For this review, take the finished solid that the model builds, in its own axes (mm). A direction names the side the tool comes from. Round coordinates to 2 decimals unless told otherwise and drop trailing zeros. Loops run counter-clockwise (first coordinate to the right, second up) from the corner with the lowest first, then second, coordinate; pieces in that order, holes last.
1) Take a section at A-A (z = -36). State the section outline as (x, y) points, then the cut area to 3 significant figures.
2) Mouldability with a two-part tool opening along X and no side actions: class faces 3 (the cylindrical face through (23.43, 1.52, -0.6)), 4 (the cylindrical face through (7.95, 1.52, -28.06)), 5 (the flat face through (6, 0, -45)) as pulls with the +X half, pulls with the -X half, needs draft (parallel to the pull), parting line crosses it, or undercut.
3) Take a section at C-C (x = 11). State the section outline as (y, z) points, then the cut area to 3 significant figures.
4) Wall thickness on L1, parallel to X at y = 0.8, z = -68; L2, parallel to X at y = 0.95, z = -84; L3, parallel to Z at x = 13.5, y = 1.45: over which ranges is each line inside the solid? List them lowest first.
5) Take a section at D-D (y = 1.85). Give the number of separate pieces and of enclosed holes in the cut face, then the cut area to 3 significant figures.
6) Tool access review of faces 1 (the cylindrical face through (16.05, 1.52, -43.94)), 2 (the flat face through (12, 1, -88)): name each direction out of +Z, -Z, +X, -X, +Y, -Y from which nothing blocks a thin tool from reaching the whole face with its end or side.
7) Take a section at B-B (z = -58.5). State the section outline as (x, y) points.
```python
from build123d import *

# Parameters (mm, degrees)
SKETCH1_W           = 24
SKETCH1_H           = 88
BOSS_EXTRUDE1_DEPTH = 3
SKETCH2_R           = 2.1
CUT_EXTRUDE1_DEPTH  = 4
SKETCH3_R           = 4.05
CUT_EXTRUDE2_DEPTH  = 4
LPATTERN1_COUNT     = 5
LPATTERN1_PITCH     = 16
SKETCH4_W           = 4.4
SKETCH4_H           = 64
CUT_EXTRUDE3_DEPTH  = 4
FILLET1_R           = 2


with BuildPart() as part:
    # Sketch1 → Boss-Extrude1 (new body)
    with BuildSketch(Plane(origin=(0, 0, 0), x_dir=(1, 0, 0), z_dir=(0, 1, 0))):
        with Locations((12, 44)):
            Rectangle(SKETCH1_W, SKETCH1_H)
    extrude(amount=BOSS_EXTRUDE1_DEPTH)

    # Sketch2 → Cut-Extrude1 (cut, through all)
    with BuildSketch(Plane(origin=(0, 3, 0), x_dir=(1, 0, 0), z_dir=(0, 1, 0))):
        with Locations((12, 84)):
            Circle(SKETCH2_R)
        with Locations((4, 84)):
            Circle(SKETCH2_R)
        with Locations((4, 76)):
            Circle(SKETCH2_R)
        with Locations((4, 68)):
            Circle(SKETCH2_R)
        with Locations((4, 52)):
            Circle(SKETCH2_R)
        with Locations((20, 52)):
            Circle(SKETCH2_R)
        with Locations((20, 68)):
            Circle(SKETCH2_R)
        with Locations((20, 76)):
            Circle(SKETCH2_R)
        with Locations((20, 84)):
            Circle(SKETCH2_R)
        with Locations((20, 4)):
            Circle(SKETCH2_R)
        with Locations((20, 12)):
            Circle(SKETCH2_R)
        with Locations((20, 20)):
            Circle(SKETCH2_R)
        with Locations((20, 36)):
            Circle(SKETCH2_R)
        with Locations((4, 36)):
            Circle(SKETCH2_R)
        with Locations((4, 20)):
            Circle(SKETCH2_R)
        with Locations((4, 12)):
            Circle(SKETCH2_R)
        with Locations((4, 4)):
            Circle(SKETCH2_R)
        with Locations((12, 4)):
            Circle(SKETCH2_R)
    extrude(amount=-CUT_EXTRUDE1_DEPTH, mode=Mode.SUBTRACT)

    # Sketch3 → Cut-Extrude2 (cut, through all)
    with BuildSketch(Plane(origin=(0, 3, 0), x_dir=(1, 0, 0), z_dir=(0, 1, 0))):
        with Locations((12, 76)):
            Circle(SKETCH3_R)
    cut_extrude2 = extrude(amount=-CUT_EXTRUDE2_DEPTH, mode=Mode.SUBTRACT)

    # LPattern1: Cut-Extrude2 ×5
    with Locations(*[(0, 0, i * LPATTERN1_PITCH) for i in range(1, LPATTERN1_COUNT)]):
        add(cut_extrude2, mode=Mode.SUBTRACT)

    # Sketch4 → Cut-Extrude3 (cut, through all)
    with BuildSketch(Plane(origin=(0, 3, 0), x_dir=(1, 0, 0), z_dir=(0, 1, 0))):
        with Locations((12, 44)):
            Rectangle(SKETCH4_W, SKETCH4_H)
    extrude(amount=-CUT_EXTRUDE3_DEPTH, mode=Mode.SUBTRACT)

    # Fillet1
    fillet1_edges = [part.edges().sort_by_distance(p)[0] for p in [
        (0, 1.5, -88),
        (24, 1.5, -88),
        (24, 1.5, 0),
        (0, 1.5, 0),
    ]]
    fillet(fillet1_edges, radius=FILLET1_R)


solid = part.part
```
Response:
1. outline: (0, 0) - (1.9, 0) - (1.9, 3) - (0, 3) - close; (6.1, 0) - (9.8, 0) - (9.8, 3) - (6.1, 3) - close; (14.2, 0) - (17.9, 0) - (17.9, 3) - (14.2, 3) - close; (22.1, 0) - (24, 0) - (24, 3) - (22.1, 3) - close
1. area: 33.6 mm2
2. face 3: pulls with the +X half
2. face 4: undercut
2. face 5: needs draft
3. outline: (0, -88) - (3, -88) - (3, -85.85) - (0, -85.85) - close; (0, -82.15) - (3, -82.15) - (3, -79.92) - (0, -79.92) - close; (0, -8.08) - (3, -8.08) - (3, -5.85) - (0, -5.85) - close; (0, -2.15) - (3, -2.15) - (3, 0) - (0, 0) - close
3. area: 26.3 mm2
4. L1: x = 0 to 1.9, 6.1 to 9.8, 14.2 to 17.9, 22.1 to 24
4. L2: x = 0 to 1.9, 6.1 to 9.9, 14.1 to 17.9, 22.1 to 24
4. L3: z = -88 to -85.47, -82.53 to -79.76, -8.24 to -5.47, -2.53 to 0
5. separate pieces: 1
5. enclosed holes: 19
5. area: 1,460 mm2
6. face 1: +Y, -Y
6. face 2: -Z, +X, -X, +Y, -Y
7. outline: (0, 0) - (8.24, 0) - (8.24, 3) - (0, 3) - close; (15.76, 0) - (24, 0) - (24, 3) - (15.76, 3) - close
